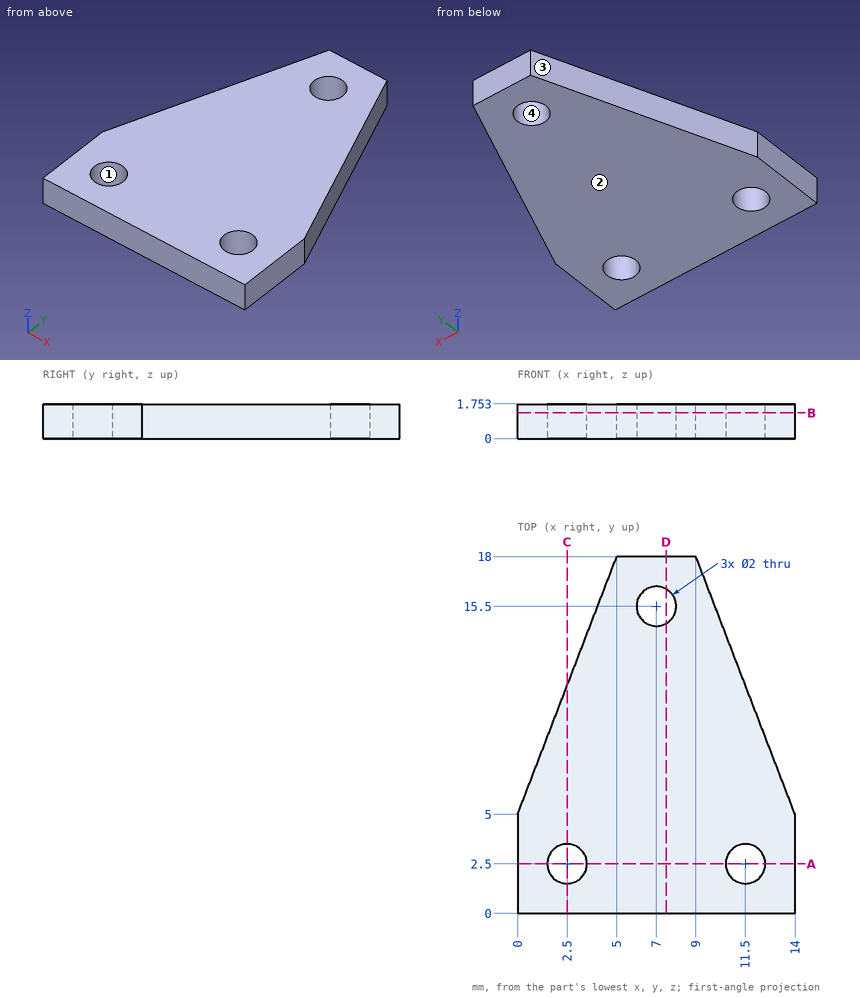
Answer from the drawing. Dimensions are ordinates in mm from the lowest x, y and z of the part. Give positions to 0.01 mm unless a question says otherwise; leave off trailing zeros. Write each loop counter-clockwise with the first axis right and the second up, starting at its lowest first coordinate (ties: lowest second). Pieces come first, ordered by that corner, then holes. Notation, with made-up numbers: (88, 25.5) - (145, 25.5) arc R15 ccw to (145, 40.5) - close; hole circle Ø6 at (-5.75, -6). An arc over 180 degrees is marked (long way). Answer in a Markdown table with one row per item. Add a question column.
Item 1: Determine the mould class of the marked faces 1, 2, 3 and 4 for opening direction X: pulls with the +X half, pulls with the -X half, needs draft (parallel to the pull), parting line crosses it, or undercut.
Item 2: Section C-C, the plane x = 2.5 is taken. Write down the section's boundary in (y, z).
Item 3: Find the intervals of material crossed by L1, parallel to X at y = 2, z = 0.35 (1 decimal); L2, parallel to X at y = 2.25, z = 0.3; L3, parallel to X at y = 15, z = 1.3 (1 decimal), in increasing order.
Item 4: Section A-A, the plane y = 2.5 is taken. Write down the section's boundary in (x, z).
Item 5: Section B-B, the plane z = 1.3 is taken. Write down the section's boundary in (x, y).
Item 6: A flat-ended cylindrical pin translates along its axis: P1, Ø1, axis at y = 12, z = 0.5, coming from the +X side. Find the tip coordinate at first contact, or state that the pin passes through.
Item 7: Section D-D, the plane x = 7.5 is taken. Write down the section's boundary in (y, z).
Recorded:
| question | item | result |
|---|---|---|
| 1 | face 1 | undercut |
| 1 | face 2 | needs draft |
| 1 | face 3 | pulls with the -X half |
| 1 | face 4 | undercut |
| 2 | outline | (0, 0) - (1.5, 0) - (1.5, 1.75) - (0, 1.75) - close; (3.5, 0) - (11.5, 0) - (11.5, 1.75) - (3.5, 1.75) - close |
| 3 | L1 | x = 0 to 1.6, 3.4 to 10.6, 12.4 to 14 |
| 3 | L2 | x = 0 to 1.53, 3.47 to 10.53, 12.47 to 14 |
| 3 | L3 | x = 3.8 to 6.1, 7.9 to 10.2 |
| 4 | outline | (0, 0) - (1.5, 0) - (1.5, 1.75) - (0, 1.75) - close; (3.5, 0) - (10.5, 0) - (10.5, 1.75) - (3.5, 1.75) - close; (12.5, 0) - (14, 0) - (14, 1.75) - (12.5, 1.75) - close |
| 5 | outline | (0, 0) - (14, 0) - (14, 5) - (9, 18) - (5, 18) - (0, 5) - close; hole circle Ø2 at (2.5, 2.5); hole circle Ø2 at (7, 15.5); hole circle Ø2 at (11.5, 2.5) |
| 6 | P1 | stops at x = 11.5 |
| 7 | outline | (0, 0) - (14.63, 0) - (14.63, 1.75) - (0, 1.75) - close; (16.37, 0) - (18, 0) - (18, 1.75) - (16.37, 1.75) - close |
